CAD build for the part. Positions are in the model's coordinates, mm. Face numbers are marked on the shaded views. A direction names the side the tool comes from. Coordinates: 2 decimals unless noted, no trailing zeros. Loops run counter-clockwise (first coordinate to the right, second up) from the corner with the lowest first, then second, coordinate; pieces in that order, holes last. Notation, with made-up numbers: (83.25, -8) -> (125.25, -8) arc R17 ccw to (125.25, 12) -> close; hole circle Ø7 at (-35, -27). An arc over 180 degrees is marked (long way). Return JSON: item names as keys, results as strings. Group by question number.
(1) Saw through at A-A on z = -3.5. Write the cut outline in (x, y), then the cut area to 3 significant figures.
(2) Flat gauge pins, fed straight in: pin 1 Ø1.6 at (x, z) = (-2.5, -1.5) entering from -Y; pin 2 Ø3 at (y, z) = (-7, -2.5) entering from +X; pin 3 Ø1 at (x, z) = (3.5, 0.5) entering from -Y. Where does each tip first touch, or does it go through?
(3) Saw through at B-B on x = -7.25. Write the cut outline in (y, z), then the cut area to 3 significant figures.
(4) Saw through at C-C on y = -7.5. Write the cut outline in (x, z).
(5) Tool access for the marked faces 1, 2, 3 and 4: list every direction of +Z, -Z, +X, -X, +Y, -Y with a clear straight run to the whole face (end or side of a thin tool).
(6) Probe L1, parallel to Z at x = -6.75, y = 10.5; L2, parallel to Z at x = 1.5, y = -5; L3, parallel to Y at x = -2.5, z = 2.75. List the from-to ranges inside material, lowest first.
(7) Saw through at D-D on x = -2.75. Write the cut outline in (y, z), then the cut area to 3 significant figures.
```python
from build123d import *

# Parameters (mm, degrees)
ESQUISSE1_R        = 14.5
BOSS_EXTRU_1_DEPTH = 1.6
ESQUISSE2_W        = 10.3
ESQUISSE2_H        = 16.2
BOSS_EXTRU_2_DEPTH = 2.4
BOSS_EXTRU_3_DEPTH = 4.45
ESQUISSE4_W        = 6
ESQUISSE4_H        = 4
BOSS_EXTRU_4_DEPTH = 5.2
ESQUISSE5_W        = 3
ESQUISSE5_H        = 1.3
BOSS_EXTRU_5_DEPTH = 1.6


with BuildPart() as part:
    # Esquisse1 → Boss.-Extru.1 (new body)
    with BuildSketch(Plane.XY):
        with Locations((-3.708152602, 4.763148131)):
            Circle(ESQUISSE1_R)
    extrude(amount=BOSS_EXTRU_1_DEPTH)

    # Esquisse2 → Boss.-Extru.2 (add)
    with BuildSketch(Plane.XY.offset(1.6)):
        with Locations((-3.708152602, 10.217759892)):
            Rectangle(ESQUISSE2_W, ESQUISSE2_H)
    extrude(amount=BOSS_EXTRU_2_DEPTH)

    # Esquisse3 → Boss.-Extru.3 (add)
    with BuildSketch(Plane(origin=(0, 0, 0), x_dir=(-1, 0, 0), z_dir=(0, 0, -1))):
        with BuildLine():
            Line((7.708152602, -4.236851869), (14.358152602, 0.763148131))
            Line((14.358152602, 0.763148131), (14.358152602, 13.763148131))
            Line((14.358152602, 13.763148131), (12.033404554, 13.763148131))
            ThreePointArc((12.033404554, 13.763148131), (3.708152602, 18.223276297), (-4.617099351, 13.763148131))
            Line((-4.617099351, 13.763148131), (-6.941847398, 13.763148131))
            Line((-6.941847398, 13.763148131), (-6.941847398, 0.763148131))
            Line((-6.941847398, 0.763148131), (-0.291847398, -4.236851869))
            Line((-0.291847398, -4.236851869), (7.708152602, -4.236851869))
        make_face()
    extrude(amount=BOSS_EXTRU_3_DEPTH)

    # Esquisse4 → Boss.-Extru.4 (add)
    with BuildSketch(Plane(origin=(0, 0, 0), x_dir=(-1, 0, 0), z_dir=(0, 0, -1))):
        with Locations((3.708152602, -6.236851869)):
            Rectangle(ESQUISSE4_W, ESQUISSE4_H)
    extrude(amount=BOSS_EXTRU_4_DEPTH)

    # Esquisse5 → Boss.-Extru.5 (add)
    with BuildSketch(Plane(origin=(0, 0, -5.2), x_dir=(-1, 0, 0), z_dir=(0, 0, -1))):
        with Locations((3.708152602, -6.236851869)):
            Rectangle(ESQUISSE5_W, ESQUISSE5_H)
    extrude(amount=BOSS_EXTRU_5_DEPTH)


solid = part.part
```
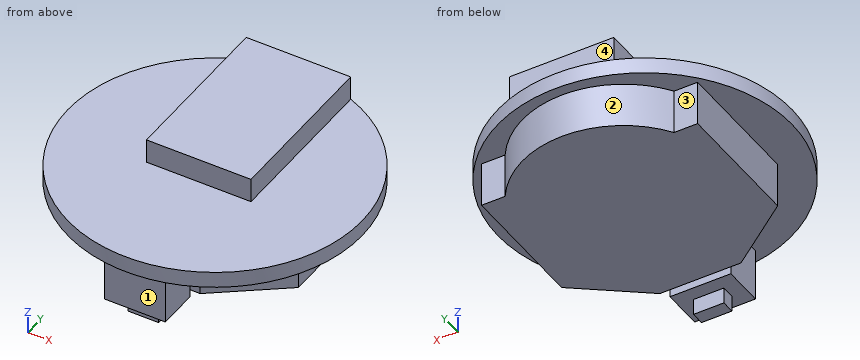
Geometry results:
{
 "1": {"outline": "(-14.36, 0.76) -> (-7.71, -4.24) -> (-6.71, -4.24) -> (-6.71, -8.24) -> (-0.71, -8.24) -> (-0.71, -4.24) -> (0.29, -4.24) -> (6.94, 0.76) -> (6.94, 13.76) -> (4.62, 13.76) arc R10 ccw to (-12.03, 13.76) -> (-14.36, 13.76) -> close", "area": "426 mm²"},
 "2": {"pin 1": "y = -8.24", "pin 2": "x = -0.71", "pin 3": "y = -8.09"},
 "3": {"outline": "(-9.3, 0) -> (-4.24, 0) -> (-4.24, -4.45) -> (17.58, -4.45) -> (17.58, 0) -> (18.82, 0) -> (18.82, 1.6) -> (18.32, 1.6) -> (18.32, 4) -> (2.12, 4) -> (2.12, 1.6) -> (-9.3, 1.6) -> close", "area": "181 mm²"},
 "4": {"outline": "(-11.45, 0) -> (-6.71, 0) -> (-6.71, -5.2) -> (-0.71, -5.2) -> (-0.71, 0) -> (4.03, 0) -> (4.03, 1.6) -> (-11.45, 1.6) -> close"},
 "5": {"face 1": "-Z, +X, -X, -Y", "face 2": "-Z, +Y", "face 3": "-Z, -X, +Y", "face 4": "+Z, +X, -X, +Y"},
 "6": {"L1": "-4.45 to 4", "L2": "0 to 1.6", "L3": "2.12 to 18.32"},
 "7": {"outline": "(-9.71, 0) -> (-8.24, 0) -> (-8.24, -5.2) -> (-6.89, -5.2) -> (-6.89, -6.8) -> (-5.59, -6.8) -> (-5.59, -5.2) -> (-4.24, -5.2) -> (-4.24, -4.45) -> (18.18, -4.45) -> (18.18, 0) -> (19.23, 0) -> (19.23, 1.6) -> (18.32, 1.6) -> (18.32, 4) -> (2.12, 4) -> (2.12, 1.6) -> (-9.71, 1.6) -> close", "area": "208 mm²"}
}
